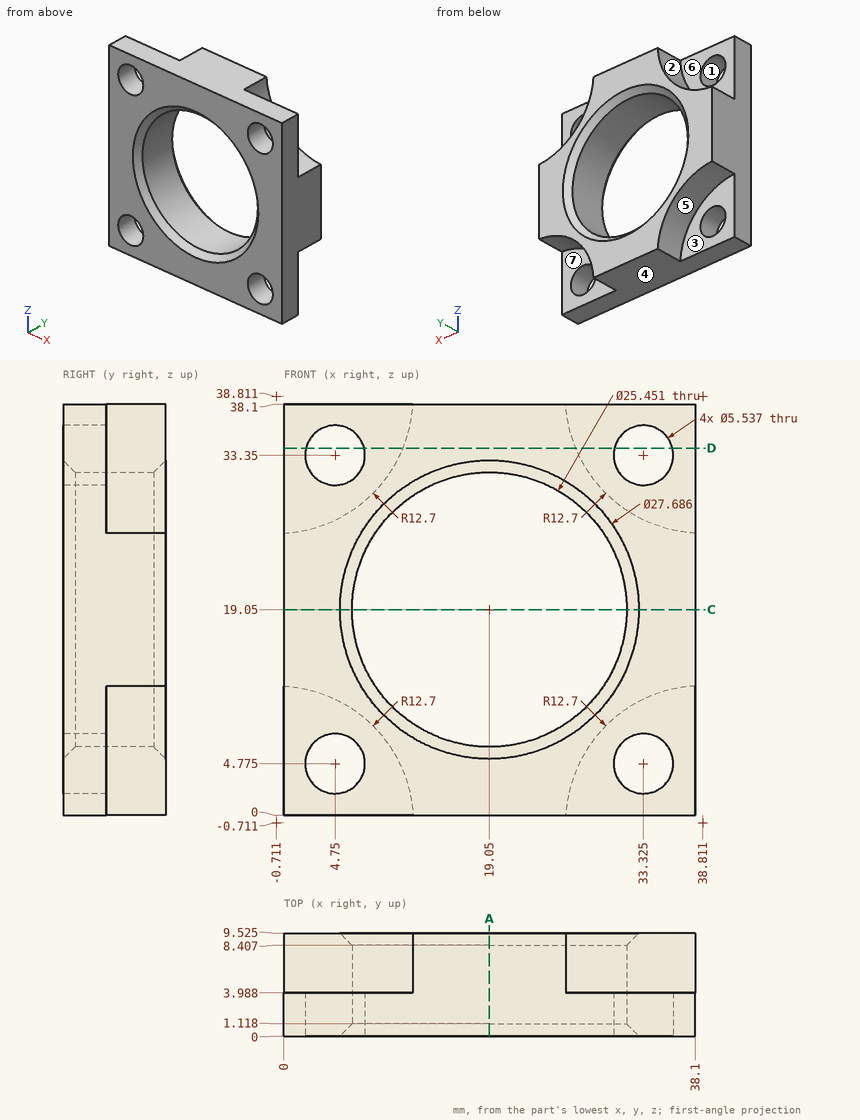
Study the drawing (mm; zero at the part's minimum x, y, z) and answer. A direction names the side the tool comes from. Round coordinates to 2 decimals unless told otherwise and drop trailing zeros. Order: outer loops, then holes, each group sorted by start corner. A loop starts at its lowest first (then second) coordinate and runs counter-clockwise, first axis right, second up. Notation, with made-up numbers: (-16, 12) - (31, 12) arc R12 ccw to (31, 23) - close; hole circle Ø1 at (46, -5.75). An arc over 180 degrees is marked (long way). Use one line per item in the form item = value. Start each with the question number.
(1) Determine the mould class of the marked faces 1, 2, 3 and 4 for opening direction Z: +Z half, -Z half, draft (parallel to the pull), parting line (faces both ways), or undercut.
(2) For the marked faces 5, 6 and 7, determine the directions among +Z, -Z, +X, -X, +Y, -Y from which every point of the face is accessible in a straight line to the end or side of a thin tool.
(3) Find the intervals of material crossed by line 1 along X through (y, z) = (7, 19.05) (1 decimal); line 2 along Z through (x, y) = (33, 1.5) (1 decimal); line 3 along Z through (x, y) = (20, 3.25), in increasing order. Write a range as from..to.
(4) Flat-ended cylindrical pins translate along their axes: pin 1 Ø7 at (x, z) = (33.32, 33.35) entering from +Y; pin 2 Ø4.5 at (x, z) = (33.32, 4.78) entering from +Y; pin 3 Ø4 at (x, z) = (8.5, 22.5) entering from -Y; pin 4 Ø1 at (y, z) = (6, 8) entering from -X. Find the tip coordinate at first contact, or state that the pin passes through.
(5) The part is cut by section A-A (x = 19.05). Give the vertices of the cut face in (y, z) (1 decimal).
(6) The part is cut by section D-D (z = 34). Give the vertices of the cut face in (x, y) (1 decimal), then the cut area to 3 significant figures.
(7) The part is cut by section C-C (z = 19.05). Give the vertices of the cut face in (x, y) (1 decimal).
Checked values:
q1.face_1 = undercut
q1.face_2 = +Z half
q1.face_3 = draft
q1.face_4 = -Z half
q2.face_5 = -Z, -X, +Y
q2.face_6 = +Z, -X, +Y
q2.face_7 = -Z, +X, +Y
q3.line_1 = 0..6.3, 31.8..38.1
q3.line_2 = 0..2, 7.5..30.6, 36.1..38.1
q3.line_3 = 0..6.36, 31.74..38.1
q4.pin_1 = 3.99
q4.pin_2 = through
q4.pin_3 = 0.74
q4.pin_4 = 8.03
q5.outline = (0, 0) - (9.5, 0) - (9.5, 5.2) - (8.4, 6.3) - (1.1, 6.3) - (0, 5.2) - close; (0, 32.9) - (1.1, 31.8) - (8.4, 31.8) - (9.5, 32.9) - (9.5, 38.1) - (0, 38.1) - close
q6.outline = (0, 0) - (2.1, 0) - (2.1, 4) - (0, 4) - close; (7.4, 0) - (30.6, 0) - (30.6, 4) - (27.1, 4) - (27.1, 9.5) - (11, 9.5) - (11, 4) - (7.4, 4) - close; (36, 0) - (38.1, 0) - (38.1, 4) - (36, 4) - close
q6.area = 198 mm^2
q7.outline = (0, 0) - (5.2, 0) - (6.3, 1.1) - (6.3, 8.4) - (5.2, 9.5) - (0, 9.5) - close; (31.8, 1.1) - (32.9, 0) - (38.1, 0) - (38.1, 9.5) - (32.9, 9.5) - (31.8, 8.4) - close
